from build123d import *

# Parameters (mm, degrees)
RESSALTO_EXTRUS_O1_DEPTH                = 40
CORTE_EXTRUS_O2_START                   = -5
CORTE_EXTRUS_O2_DEPTH                   = 25
CORTE_EXTRUS_O3_DEPTH                   = 25
ESBO_O4_R                               = 30
ESBO_O4_R_2                             = 5
CORTE_EXTRUS_O4_DEPTH                   = 10
BROCA_DE_ROSQUEAR_PARA_TARRAXA_DE_M31_D = 2.5
BROCA_DE_ROSQUEAR_PARA_TARRAXA_DE_M32_D = 2.5


with BuildPart() as part:
    # Esboço1 → Ressalto-extrusão1 (new body)
    with BuildSketch(Plane(origin=(0, 0, 0), x_dir=(1, 0, 0), z_dir=(0, 1, 0))):
        Polygon((146.682207566, -60.757759733), (146.682207566, 60.757759733), (60.757759733, 146.682207566), (-60.757759733, 146.682207566), (-146.682207566, 60.757759733), (-146.682207566, -60.757759733), (-60.757759733, -146.682207566), (60.757759733, -146.682207566), align=None)
    extrude(amount=RESSALTO_EXTRUS_O1_DEPTH)

    # Esboço2 → Corte-extrusão2 (cut)
    with BuildSketch(Plane(origin=(0, 40, 0), x_dir=(1, 0, 0), z_dir=(0, 1, 0)).offset(CORTE_EXTRUS_O2_START)):
        Polygon((120.710678119, 50), (50, 120.710678119), (-50, 120.710678119), (-120.710678119, 50), (-120.710678119, -50), (-50, -120.710678119), (50, -120.710678119), (120.710678119, -50), align=None)
    extrude(amount=-CORTE_EXTRUS_O2_DEPTH, mode=Mode.SUBTRACT)

    # Esboço3 → Corte-extrusão3 (cut)
    with BuildSketch(Plane(origin=(0, 40, 0), x_dir=(1, 0, 0), z_dir=(0, 1, 0))):
        Polygon((120.710678119, 50), (50, 120.710678119), (-50, 120.710678119), (-120.710678119, 50), (-120.710678119, -50), (-50, -120.710678119), (50, -120.710678119), (120.710678119, -50), align=None)
    extrude(amount=-CORTE_EXTRUS_O3_DEPTH, mode=Mode.SUBTRACT)

    # Esboço4 → Corte-extrusão4 (cut)
    with BuildSketch(Plane(origin=(0, 10, 0), x_dir=(1, 0, 0), z_dir=(0, 1, 0))):
        with Locations(Location((0, 0, 0), (0, 0, 270))):
            Circle(ESBO_O4_R)
        with Locations(Location((-74.266400318, 16.749004229, 0), (0, 0, 270))):
            Circle(ESBO_O4_R_2)
        with Locations(Location((-59.761337168, 8.374502115, 0), (0, 0, 270))):
            Circle(ESBO_O4_R_2)
        with Locations(Location((-59.761337168, -8.374502115, 0), (0, 0, 270))):
            Circle(ESBO_O4_R_2)
        with Locations(Location((-74.266400318, -16.749004229, 0), (0, 0, 270))):
            Circle(ESBO_O4_R_2)
        with Locations(Location((-88.771463469, -8.374502115, 0), (0, 0, 270))):
            Circle(ESBO_O4_R_2)
        with Locations(Location((-88.771463469, 8.374502115, 0), (0, 0, 270))):
            Circle(ESBO_O4_R_2)
        with Locations(Location((-74.266400318, 0, 0), (0, 0, 270))):
            Circle(ESBO_O4_R_2)
        with Locations(Location((74.266400318, 0, 0), (0, 0, 90))):
            Circle(ESBO_O4_R_2)
        with Locations(Location((88.771463469, 8.374502115, 0), (0, 0, 90))):
            Circle(ESBO_O4_R_2)
        with Locations(Location((88.771463469, -8.374502115, 0), (0, 0, 90))):
            Circle(ESBO_O4_R_2)
        with Locations(Location((74.266400318, -16.749004229, 0), (0, 0, 90))):
            Circle(ESBO_O4_R_2)
        with Locations(Location((59.761337168, -8.374502115, 0), (0, 0, 90))):
            Circle(ESBO_O4_R_2)
        with Locations(Location((59.761337168, 8.374502115, 0), (0, 0, 90))):
            Circle(ESBO_O4_R_2)
        with Locations(Location((74.266400318, 16.749004229, 0), (0, 0, 90))):
            Circle(ESBO_O4_R_2)
        with BuildLine():
            ThreePointArc((-71.17306789, 67.045187012), (-77.704390833, 39.454208035), (-50.081737205, 33.058169667))
            add(Edge.make_bspline(
                [(-50.081737205, 33.058169667), (0, 55.749902863), (50.081737205, 33.058169667)],
                knots=[0, 0, 0, 1, 1, 1], degree=2))
            ThreePointArc((50.081737205, 33.058169667), (77.704390833, 39.454208035), (71.17306789, 67.045187012))
            add(Edge.make_bspline(
                [(-71.17306789, 67.045187012), (0, 101.762885517), (71.17306789, 67.045187012)],
                knots=[0, 0, 0, 1, 1, 1], degree=2))
        make_face()
        with BuildLine():
            ThreePointArc((-71.17306789, -67.045187012), (-77.704390833, -39.454208035), (-50.081737205, -33.058169667))
            add(Edge.make_bspline(
                [(-50.081737205, -33.058169667), (0, -55.749902863), (50.081737205, -33.058169667)],
                knots=[0, 0, 0, 1, 1, 1], degree=2))
            ThreePointArc((50.081737205, -33.058169667), (77.704390833, -39.454208035), (71.17306789, -67.045187012))
            add(Edge.make_bspline(
                [(-71.17306789, -67.045187012), (0, -101.762885517), (71.17306789, -67.045187012)],
                knots=[0, 0, 0, 1, 1, 1], degree=2))
        make_face()
    extrude(amount=-CORTE_EXTRUS_O4_DEPTH, mode=Mode.SUBTRACT)

    # Broca de rosquear para tarraxa de M31 (through all)
    with Locations(Plane(origin=(103.719983649, 0, 103.719983649), x_dir=(0.7071067811865479, 0, -0.7071067811865472), z_dir=(0.7071067811865472, 0, 0.7071067811865479))):
        with Locations((-20, 20), (20, 20)):
            Hole(BROCA_DE_ROSQUEAR_PARA_TARRAXA_DE_M31_D / 2)

    # Broca de rosquear para tarraxa de M32 (through all)
    with Locations(Plane(origin=(-103.719983649, 0, 103.719983649), x_dir=(0.7071067811865476, 0, 0.7071067811865476), z_dir=(-0.7071067811865476, 0, 0.7071067811865476))):
        with Locations((-20, 20), (20, 20)):
            Hole(BROCA_DE_ROSQUEAR_PARA_TARRAXA_DE_M32_D / 2)


solid = part.part
For this review, take the finished solid that the model builds, in its own axes (mm). A direction names the side the tool comes from. Round coordinates to 2 decimals unless told otherwise and drop trailing zeros. Loops run counter-clockwise (first coordinate to the right, second up) from the corner with the lowest first, then second, coordinate; pieces in that order, holes last. Notation, with made-up numbers: (-26.5, 50.25) - (-20.5, 50.25) arc R18 cw to (-20.5, 67.25) - close; hole circle Ø2 at (87.5, 20.5). An arc over 180 degrees is marked (long way). Put each result on its own line as item: value. Start each with the question number.
1. Mouldability with a two-part tool opening along X and no side actions: class faces 3 (the cylindrical face through (107.71, 20.38, 81.11)), 4 (the flat face through (120.711, 25, 1)) as +X half, -X half, draft (parallel to the pull), parting line (faces both ways), or undercut.
2. Consider section A-A on z = 0. State the section outline as (x, y) points.
3. For faces 1 (the flat face through (-84.86, 25.21, -85.85)), 2 (the cylindrical face through (81.41, 20.05, -107.93)), list the 3-axis set-ups (+Z, -Z, +X, -X, +Y, -Y) from which the entire face can be reached by the end or side of a thin tool; tool diameter is ignored.
4. Insertion check: P1, Ø11.5, axis at x = 74.27, z = -16.75, coming from the +Y side; P2, Ø2, axis at x = 86, y = 15.5, coming from the -Z side; P3, Ø4, axis at y = 11, z = -113, coming from the +X side. Each pin has a flat end and moves straight along its axis. Give the tip position at first contact, or say it passes through.
5. For probe 1 along X at (y, z) = (7.5, 0); probe 2 along Z at (x, y) = (-21.5, 23), list the stretches that pass through material, from the lowest coordinate up. Write a range as [from, to].
6. Consider section B-B on x = 0. State how many separate pieces and enclosed holes the cut face has, plus the area to 3 significant figures.
Result sheet:
1. face 3: undercut
1. face 4: undercut
2. outline: (-146.68, 0) - (-79.27, 0) - (-79.27, 10) - (-120.71, 10) - (-120.71, 40) - (-146.68, 40) - close; (-69.27, 0) - (-30, 0) - (-30, 10) - (-69.27, 10) - close; (30, 0) - (69.27, 0) - (69.27, 10) - (30, 10) - close; (79.27, 0) - (146.68, 0) - (146.68, 40) - (120.71, 40) - (120.71, 10) - (79.27, 10) - close
3. face 1: +Y
3. face 2: none
4. P1: y = 10
4. P2: z = -122.44
4. P3: x = 96.44
5. probe 1: [-146.68, -79.27], [-69.27, -30], [30, 69.27], [79.27, 146.68]
5. probe 2: [-146.68, -120.71], [120.71, 146.68]
6. separate pieces: 4
6. enclosed holes: 0
6. area: 3,090 mm^2
